Autodesk Fusion 360 part; units mm, degrees
sketch "Sketch1" plane through (0, 0, 0) normal (0, 0, 1) x (1, 0, 0)
  circle A0 centre (0, 0) radius 11
  circle A1 centre (0, 0) radius 13.5
  circle A2 centre (0, 0) radius 45 construction
  circle A3 centre (-0.0744, 35.9127) radius 9
  arc A4 (-13.3245, 2.1699) -> (-8.9923, 34.7002) centre (-571.0597, 92.9983) ccw
  line L0 (8.8488, 34.7395) -> (13.3741, 1.8396)
  line L1 (-3.5385, 41.9127) -> (-7.0026, 35.9127)
  line L2 (-7.0026, 35.9127) -> (-3.5385, 29.9127)
  line L3 (-3.5385, 29.9127) -> (3.3897, 29.9127)
  line L4 (3.3897, 29.9127) -> (6.8538, 35.9127)
  line L5 (6.8538, 35.9127) -> (3.3897, 41.9127)
  line L6 (3.3897, 41.9127) -> (-3.5385, 41.9127)
  line L7 (-27.6, -24.0208) -> (-24.1359, -18.0208)
  line L8 (-34.5282, -24.0208) -> (-27.6, -24.0208)
  line L9 (-24.1359, -18.0208) -> (-27.6, -12.0208)
  circle A5 centre (-31.0641, -18.0208) radius 9
  line L10 (-34.5282, -12.0208) -> (-37.9923, -18.0208)
  arc A6 (4.783, -12.6243) -> (-25.5551, -25.1377) centre (204.991, -541.0514) ccw
  line L11 (-27.6, -12.0208) -> (-34.5282, -12.0208)
  line L12 (-34.5097, -9.7065) -> (-8.2801, 10.6625)
  line L13 (-37.9923, -18.0208) -> (-34.5282, -24.0208)
  line L14 (34.6026, -11.8919) -> (27.6744, -11.8919)
  line L15 (38.0667, -17.8919) -> (34.6026, -11.8919)
  line L16 (27.6744, -11.8919) -> (24.2103, -17.8919)
  circle A7 centre (31.1385, -17.8919) radius 9
  line L17 (27.6744, -23.8919) -> (34.6026, -23.8919)
  arc A8 (8.5414, 10.4544) -> (34.5474, -9.5625) centre (366.0688, 448.0531) ccw
  line L18 (24.2103, -17.8919) -> (27.6744, -23.8919)
  line L19 (25.6609, -25.0331) -> (-5.0939, -12.5021)
  line L20 (34.6026, -23.8919) -> (38.0667, -17.8919)
  point P0 (-0.0744, 35.9127)
  point P1 (-31.0641, -18.0208)
  point P2 (31.1385, -17.8919)
  dimension "d1" = 22
  dimension "d2" = 27
  dimension "d4" = 90
  dimension "d5" = 18
  dimension "d6" = 6
  dimension "d8" = 360
extrude "Extrude1" add sketch "Sketch1" along normal blind 5
The listing builds one solid part. Answer for the finished solid, in the listing's coordinates (mm). A direction names the side the tool comes from. Round coordinates to 2 decimals unless told otherwise and drop trailing zeros. Order: outer loops, then holes, each group sorted by start corner. A loop starts at its lowest first (then second) coordinate and runs counter-clockwise, first axis right, second up. Notation, with made-up numbers: (-13, 21.5) - (39, 21.5) arc R27 cw to (39, 39.5) - close; hole circle Ø10 at (35, -7). An arc over 180 degrees is marked (long way). Put each result on its own line as item: value. Start each with the question number.
(1) Find section B-B (z = 3.85). Give the vertices of the cut face in (x, y), plus the area to 3 significant figures.
(2) Find section C-C (y = 0). Give the vertices of the cut face in (x, z).
(3) Given P1, Ø2, axis at x = -9, z = 3, coming from the -Y side; P2, Ø12, axis at x = -31, y = 4.5, coming from the -Z side; P3, Ø1.5, axis at x = -1, z = 3, coming from the +Y side; P4, Ø3, axis at y = 30, z = 2, coming from the -X side, each flat-ended and moving along its own axis, determine where each tip first touches the part or whether it passes through.
(4) Find section D-D (x = 23). Give the vertices of the cut face in (y, z), plus the area to 3 significant figures.
(5) Straight lines are drawn through the part: probe 1 along X at (y, z) = (-13, 0.65); probe 2 along Y at (x, z) = (2, 1.95); probe 3 along Y at (x, z) = (0, 1.6). For each, find the intervals that lie inside material, in ascending order. Write a range as from..to.
(6) For faces 4 (the flat face through (-36.236, -14.979, 2.465)), 5 (the cylindrical face through (23.648, -1.465, 2.465)), 6 (the flat face through (12.94, -19.85, 2.46)), determine the directions among +Z, -Z, +X, -X, +Y, -Y from which every point of the face is accessible in a straight line to the end or side of a thin tool.
(7) Find section A-A (x = 2.5). Give the vertices of the cut face in (y, z).
(8) Determine the mould class of faces 1 (the flat face through (-6, -10, 0)), 2 (the flat face through (36.31, -20.934, 2.465)), 3 (the flat face through (10.72, 21.13, 2.46)) for opening direction X: released by +X, released by -X, zero draft, split by the parting line, or undercut.
Reply:
1. outline: (-34.51, -9.71) arc R9 ccw (long way) to (-25.56, -25.14) arc R565.08 cw to (-0.15, -14.52) - (25.66, -25.03) arc R9 ccw (long way) to (34.55, -9.56) arc R565.08 cw to (12.65, 7.13) - (8.85, 34.74) arc R9 ccw (long way) to (-8.99, 34.7) arc R565.08 cw to (-12.5, 7.39) - close; hole (-37.99, -18.02) - (-34.53, -24.02) - (-27.6, -24.02) - (-24.14, -18.02) - (-27.6, -12.02) - (-34.53, -12.02) - close; hole circle Ø22 at (0, 0); hole (-7, 35.91) - (-3.54, 29.91) - (3.39, 29.91) - (6.85, 35.91) - (3.39, 41.91) - (-3.54, 41.91) - close; hole (24.21, -17.89) - (27.67, -23.89) - (34.6, -23.89) - (38.07, -17.89) - (34.6, -11.89) - (27.67, -11.89) - close
1. area: 1,730 mm^2
2. outline: (-22.01, 0) - (-11, 0) - (-11, 5) - (-22.01, 5) - close; (11, 0) - (21.73, 0) - (21.73, 5) - (11, 5) - close
3. P1: y = -18.46
3. P2: through
3. P3: y = 44.91
3. P4: x = -9.67
4. outline: (-23.95, 0) - (-0.97, 0) - (-0.97, 5) - (-23.95, 5) - close
4. area: 115 mm^2
5. probe 1: -38.53..-35.09, -27.03..27.03, 35.24..38.69
5. probe 2: -15.39..-10.82, 10.82..29.91, 41.91..44.67
5. probe 3: -14.58..-11, 11..29.91, 41.91..44.91
6. face 4: +Z, -Z
6. face 5: +Z, -Z, +X, +Y
6. face 6: +Z, -Z, -Y
7. outline: (-15.6, 0) - (-10.71, 0) - (-10.71, 5) - (-15.6, 5) - close; (10.71, 0) - (29.91, 0) - (29.91, 5) - (10.71, 5) - close; (41.91, 0) - (44.54, 0) - (44.54, 5) - (41.91, 5) - close
8. face 1: zero draft
8. face 2: undercut
8. face 3: released by +X
